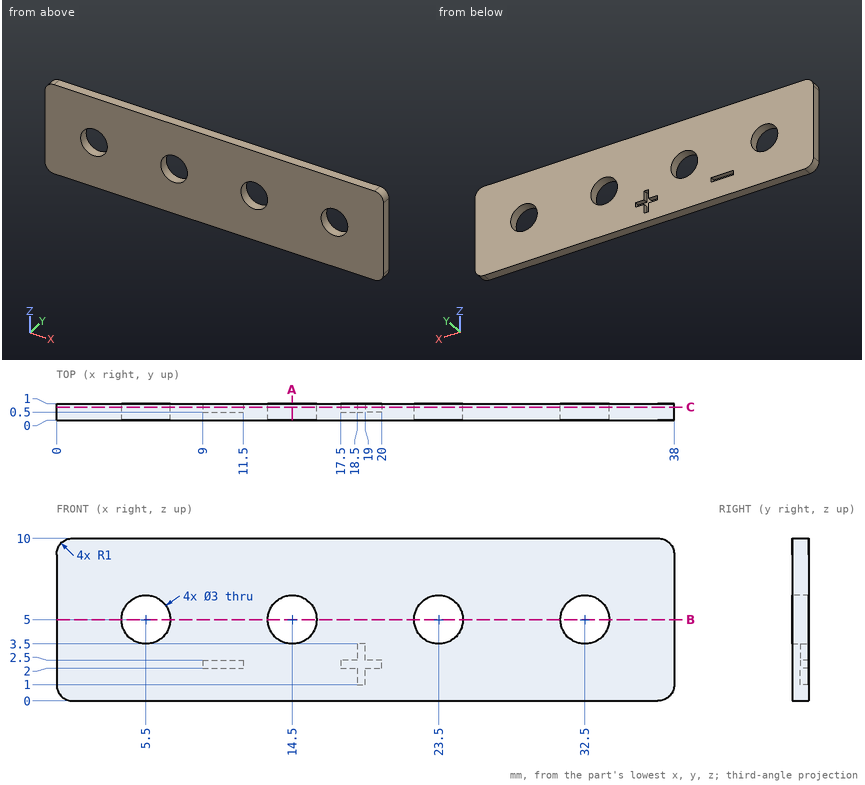
The drawing under review shows one solid part. Ordinate dimensions are in mm from its lowest x, y, z. Give positions to 0.01 mm unless a question says otherwise; leave off trailing zeros. Order: outer loops, then holes, each group sorted by start corner. A loop starts at its lowest first (then second) coordinate and runs counter-clockwise, first axis right, second up. Notation, with made-up numbers: M -27.75,70.25 L 21.25,70.25 A31 ccw 21.25,97.25 Z; hole C 29,74 d11. An arc over 180 degrees is marked long. Answer in a Markdown table with one row per item. Add a question column.
1. Add section B-B on z = 5. State the section outline as (x, y) points.
2. Add section A-A on x = 14.5. State the section outline as (y, z) points, plus the area to 3 significant figures.
3. To check wall thickness, follow line 1 along X through (y, z) = (0.3, 5); line 2 along X through (y, z) = (0.6, 4.5); line 3 along Z through (x, y) = (32, 0.95). State the ranges of each line that lie inside material, in increasing order.
4. Add section C-C on y = 0.8. State the section outline as (x, z) points.
The answers:
| question | item | result |
|---|---|---|
| 1 | outline | M 0,0 L 4,0 L 4,1 L 0,1 Z; M 7,0 L 13,0 L 13,1 L 7,1 Z; M 16,0 L 22,0 L 22,1 L 16,1 Z; M 25,0 L 31,0 L 31,1 L 25,1 Z; M 34,0 L 38,0 L 38,1 L 34,1 Z |
| 2 | outline | M 0,0 L 1,0 L 1,3.5 L 0,3.5 Z; M 0,6.5 L 1,6.5 L 1,10 L 0,10 Z |
| 2 | area | 7.00 mm2 |
| 3 | line 1 | 0 to 4, 7 to 13, 16 to 22, 25 to 31, 34 to 38 |
| 3 | line 2 | 0 to 4.09, 6.91 to 13.09, 15.91 to 22.09, 24.91 to 31.09, 33.91 to 38 |
| 3 | line 3 | 0 to 3.59, 6.41 to 10 |
| 4 | outline | M 0,1 A1 ccw 1,0 L 37,0 A1 ccw 38,1 L 38,9 A1 ccw 37,10 L 1,10 A1 ccw 0,9 Z; hole C 5.5,5 d3; hole M 9,2 L 11.5,2 L 11.5,2.5 L 9,2.5 Z; hole C 14.5,5 d3; hole M 17.5,2 L 18.5,2 L 18.5,1 L 19,1 L 19,2 L 20,2 L 20,2.5 L 19,2.5 L 19,3.5 L 18.5,3.5 L 18.5,2.5 L 17.5,2.5 Z; hole C 23.5,5 d3; hole C 32.5,5 d3 |
